```python
from build123d import *

# Parameters (mm, degrees)
SKETCH3_W           = 250
SKETCH3_H           = 125
BOSS_EXTRUDE1_DEPTH = 5
SKETCH10_W          = 5
SKETCH10_H          = 25
CUT_EXTRUDE4_DEPTH  = 6
SKETCH11_W          = 240
SKETCH11_H          = 5
CUT_EXTRUDE5_DEPTH  = 2.5


with BuildPart() as part:
    # Sketch3 → Boss-Extrude1 (new body)
    with BuildSketch(Plane(origin=(0, 0, 0), x_dir=(1, 0, 0), z_dir=(0, 1, 0))):
        with Locations((125, 62.5)):
            Rectangle(SKETCH3_W, SKETCH3_H)
    extrude(amount=BOSS_EXTRUDE1_DEPTH)

    # Sketch10 → Cut-Extrude4 (cut, through all)
    with BuildSketch(Plane(origin=(0, 5, 0), x_dir=(1, 0, 0), z_dir=(0, 1, 0))):
        with Locations((2.5, 87.5)):
            Rectangle(SKETCH10_W, SKETCH10_H)
        with Locations((247.5, 37.5)):
            Rectangle(SKETCH10_W, SKETCH10_H)
        with Locations((2.5, 37.5)):
            Rectangle(SKETCH10_W, SKETCH10_H)
        with Locations((247.5, 87.5)):
            Rectangle(SKETCH10_W, SKETCH10_H)
    extrude(amount=-CUT_EXTRUDE4_DEPTH, mode=Mode.SUBTRACT)

    # Sketch11 → Cut-Extrude5 (cut)
    with BuildSketch(Plane.XZ):
        with Locations((125, -12.5)):
            Rectangle(SKETCH11_W, SKETCH11_H)
    extrude(amount=-CUT_EXTRUDE5_DEPTH, mode=Mode.SUBTRACT)


solid = part.part
```
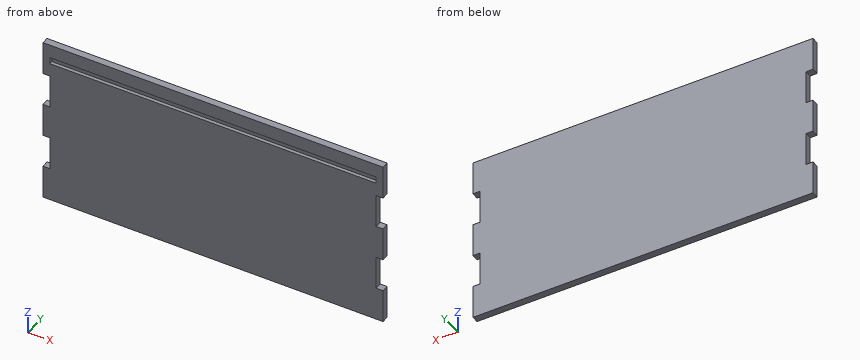
CAD build for the part. Positions are in the model's coordinates, mm. Coordinates: 2 decimals unless noted, no trailing zeros. Order: outer loops, then holes, each group sorted by start corner. A loop starts at its lowest first (then second) coordinate and runs counter-clockwise, first axis right, second up. Notation, with made-up numbers: M -22,-15.5 L -17,-15.5 A17 cw -17,8.5 Z; hole C 76.25,-21 d8. An arc over 180 degrees is marked long. Answer as CSV lines item,"result".
1) Cut at C-C (x = 105.5). List the corners of the cut face in (y, z).
Verdict:
outline,"M 0,-125 L 5,-125 L 5,0 L 0,0 L 0,-10 L 2.5,-10 L 2.5,-15 L 0,-15 Z"
2) Cut at A-A (y = 0.85). List the corners of the cut face in (x, z).
Verdict:
outline,"M 0,-125 L 250,-125 L 250,-100 L 245,-100 L 245,-75 L 250,-75 L 250,-50 L 245,-50 L 245,-25 L 250,-25 L 250,0 L 0,0 L 0,-25 L 5,-25 L 5,-50 L 0,-50 L 0,-75 L 5,-75 L 5,-100 L 0,-100 Z; hole M 5,-15 L 245,-15 L 245,-10 L 5,-10 Z"
3) Flat gauge pins, fed straight in: P1, Ø2.5, axis at x = 248, y = 3.5, coming from the +Z side; P2, Ø1.5, axis at y = 1.5, z = -49, coming from the +X side; P3, Ø3, axis at y = 0.5, z = -34, coming from the -X side. Where does each tip first touch, or does it go through?
Verdict:
P1,"z = 0"
P2,"x = 245"
P3,"x = 5"
4) Cut at D-D (z = -47). List the corners of the cut face in (x, y), then the cut area to 3 significant figures.
Verdict:
outline,"M 5,0 L 245,0 L 245,5 L 5,5 Z"
area,"1,200 mm2"
5) Drill centre lines: L1, parallel to Z at x = 238, y = 0.4; L2, parallel to X at y = 0.6, z = -88; L3, parallel to Y at x = 93, z = -13. Where is each one in solid material? Low to high. Write a range as from..to.
Verdict:
L1,"-125..-15, -10..0"
L2,"5..245"
L3,"2.5..5"
6) Cut at B-B (z = -12.5). List the corners of the cut face in (x, y).
Verdict:
outline,"M 0,0 L 5,0 L 5,2.5 L 245,2.5 L 245,0 L 250,0 L 250,5 L 0,5 Z"
